Read the model definition and answer for the solid it produces. Units are mm, in the model's axes. A direction names the side the tool comes from. Round coordinates to 2 decimals unless told otherwise and drop trailing zeros. Order: outer loops, then holes, each group sorted by start corner. A loop starts at its lowest first (then second) coordinate and runs counter-clockwise, first axis right, second up. Notation, with made-up numbers: (30.25, -11) - (60.25, -11) arc R15 ccw to (60.25, 14) - close; hole circle Ø2 at (30, 60.5). An arc over 180 degrees is marked (long way). Put each result on its own line as item: value. Start each with the question number.
Q1. Section B-B on z = 398.5 is taken. Give the vertices of the cut face in (x, y) (3 decimals).
Q2. For a pull along X with two mould halves and no side action, classify faces 1 (the face through (-10, 0, 1200)), 2 (the face through (-9.525, 0, 591)), 3 (the face through (12.7, 0, 591)) as pulls with the +X half, pulls with the -X half, needs draft (parallel to the pull), parting line crosses it, or undercut.
Q3. Each of these flat-tipped pins is pushed along its axis until it touches: pin 1 Ø8 at (x, z) = (8, 347.5) entering from +Y; pin 2 Ø6 at (x, y) = (-7.5, 17.5) entering from +Z; pin 3 Ø6 at (x, y) = (10, -15) entering from +Z. Where does it stop, or does it pass through?
Q4. Section A-A on y = 4 is taken. Give the vertices of the cut face in (x, z) (3 decimals).
Q5. Find the intervals of material crossed by line 1 along Y through (x, z) = (7.25, 923.5); line 2 along X through (y, z) = (-14, 73.5) (3 decimals); line 3 along Y through (x, z) = (-0.25, 358.5) (3 decimals), in increasing order. Write a range as from..to.
Q6. Which of the six approach directions +Z, -Z, +X, -X, +Y, -Y give full straight-line access (tool end or side, diameter ignored) to faces 4 (the face through (9.525, 0, 591)), 5 (the face through (-12.7, 0, 591))?
Autodesk Inventor part; units mm, degrees
ref_plane "Start Plane" through (0, 0, -25.4) normal (0, 0, 1) x (1, 0, 0)
ref_plane "End Plane" through (0, 0, 1225.4) normal (0, 0, 1) x (1, 0, 0)
ref_plane "Work Plane4" through (0, -25.4, 1225.4) normal (0, 0.7071, 0.7071) x (1, 0, 0)
ref_plane "Start Plane" through (0, 0, -25.4) normal (0, 0, 1) x (1, 0, 0)
ref_plane "End Plane" through (0, 0, 1225.4) normal (0, 0, 1) x (1, 0, 0)
sketch "Sketch" plane through (0, 0, 0) normal (0, 0, 1) x (1, 0, 0)
  line L0 (-12.7, -19.05) -> (-12.7, 19.05)
  line L1 (-6.35, 25.4) -> (6.35, 25.4)
  line L2 (12.7, 19.05) -> (12.7, -19.05)
  line L3 (6.35, -25.4) -> (-6.35, -25.4)
  arc A0 (-12.7, -19.05) -> (-6.35, -25.4) centre (-6.35, -19.05) ccw
  arc A1 (-6.35, 25.4) -> (-12.7, 19.05) centre (-6.35, 19.05) ccw
  arc A2 (12.7, 19.05) -> (6.35, 25.4) centre (6.35, 19.05) ccw
  arc A3 (6.35, -25.4) -> (12.7, -19.05) centre (6.35, -19.05) ccw
  arc A4 (-6.35, 22.225) -> (-9.525, 19.05) centre (-6.35, 19.05) ccw
  line L4 (-6.35, 22.225) -> (6.35, 22.225)
  arc A5 (9.525, 19.05) -> (6.35, 22.225) centre (6.35, 19.05) ccw
  line L5 (9.525, 19.05) -> (9.525, -19.05)
  arc A6 (6.35, -22.225) -> (9.525, -19.05) centre (6.35, -19.05) ccw
  line L6 (6.35, -22.225) -> (-6.35, -22.225)
  arc A7 (-9.525, -19.05) -> (-6.35, -22.225) centre (-6.35, -19.05) ccw
  line L7 (-9.525, -19.05) -> (-9.525, 19.05)
  line L8 (0, 37.4012) -> (0, -37.4012) construction
  line L9 (-19.6212, 0) -> (19.6212, 0) construction
  dimension "d10" = 50.8
  dimension "d11" = 25.4
  dimension "d12" = 3.175
  dimension "d15" = 25.4
  dimension "d16" = 12.7
  dimension "d17" = 6.35
extrude "Body" add sketch "Sketch" along normal up to surface (1250.8 mm away) from surface at -25.4
sketch "Sketch3" plane through (0, 0, 0) normal (0, 0, 1) x (1, 0, 0)
  line L0 (0, 0) -> (10, 0)
ref_plane "Work Plane3" through (0, 0, 0) normal (0, -1, 0) x (1, 0, 0)
ref_plane "Work Plane4" through (0, -25.4, 1225.4) normal (0, 0.7071, 0.7071) x (1, 0, 0)
split "Split1" plane through (0, -25.4, 1225.4) removes the side toward (0, 0.7071, 0.7071)
ref_plane "Work Plane5" through (0, 0, 0) normal (0, 0.7071, -0.7071) x (1, 0, 0)
split "Split2" plane through (0, 0, 0) removes the side toward (0, 0.7071, -0.7071)
sketch "Sketch4" plane through (0, 0, 0) normal (0, -1, 0) x (1, 0, 0)
  line L0 (-2, -25.4) -> (12, -25.4)
  line L1 (-2, 1225.4) -> (12, 1225.4)
  dimension "d19" = 1250.8
equation "\"d10\" = G_H"
equation "\"d11\" = G_W"
equation "\"d12\" = G_T"
equation "\"d15\" = 0.5 * d10"
equation "\"d16\" = 0.5 * d11"
equation "\"d17\" = G_IR"
equation "\"d3\" = G_L"
equation "\"G_W\" = 25.4"
equation "\"G_H\" = 50.8"
equation "\"G_T\" = 3.175"
equation "\"G_IR\" = 6.35"
equation "\"G_L\" = d19"
equation "\"G_OFFSET_START\" = 25.4"
equation "\"G_OFFSET_END\" = 25.4"
equation "\"d13\" = -G_OFFSET_START"
equation "\"d14\" = G_OFFSET_END + B_L"
equation "\"B_L\" = 1200"
properties part number "AISC - 2 x 1 x 1/8 - 49.244" material "Steel, Wrought"
Findings:
1. outline: (-12.7, -19.05) arc R6.35 ccw to (-6.35, -25.4) - (6.35, -25.4) arc R6.35 ccw to (12.7, -19.05) - (12.7, 19.05) arc R6.35 ccw to (6.35, 25.4) - (-6.35, 25.4) arc R6.35 ccw to (-12.7, 19.05) - close; hole (-9.525, -19.05) arc R3.175 ccw to (-6.35, -22.225) - (6.35, -22.225) arc R3.175 ccw to (9.525, -19.05) - (9.525, 19.05) arc R3.175 ccw to (6.35, 22.225) - (-6.35, 22.225) arc R3.175 ccw to (-9.525, 19.05) - close
2. face 1: needs draft
2. face 2: undercut
2. face 3: pulls with the +X half
3. pin 1: y = 25.4
3. pin 2: z = 1184.71
3. pin 3: z = 1218
4. outline: (-12.7, 4) - (-9.525, 4) - (-9.525, 1196) - (-12.7, 1196) - close; (9.525, 4) - (12.7, 4) - (12.7, 1196) - (9.525, 1196) - close
5. line 1: -25.34..-22.09, 22.09..25.34
5. line 2: -12.7..-9.525, 9.525..12.7
5. line 3: -25.4..-22.225, 22.225..25.4
6. face 4: +Z, -Z
6. face 5: +Z, -Z, -X, +Y, -Y
